Autodesk Inventor part; units mm, degrees
ref_plane "YZ Plane" through (0, 0, 0) normal (1, 0, 0) x (0, 1, 0)
ref_plane "XZ Plane" through (0, 0, 0) normal (0, 1, 0) x (-1, 0, 0)
ref_plane "XY Plane" through (0, 0, 0) normal (0, 0, 1) x (1, 0, 0)
sketch "Sketch1" plane through (0, 0, 0) normal (0, 0, 1) x (1, 0, 0)
  arc A0 (21.0123, -15.4044) -> (-20.0568, -16.8099) centre (-0.0744, 0.0265) ccw
  arc A1 (-1.3604, -38.9999) -> (3.8767, -38.8206) centre (1.1877, -36.8529) ccw
  line L0 (-1.3604, -38.9999) -> (-20.0568, -16.8099)
  line L1 (3.8767, -38.8206) -> (21.0123, -15.4044)
  point P0 (0, 0)
ref_plane "Work Plane1" through (21.0123, -15.4044, 0) normal (0.5906, 0.807, 0) x (-0.807, 0.5906, 0)
sketch "Sketch2" plane through (21.0123, -15.4044, 0) normal (0.5906, 0.807, 0) x (-0.807, 0.5906, 0)
  line L0 (1.0661, 2.0494) -> (-0.4231, 2.0494)
  line L1 (-0.4231, 2.0494) -> (-0.4231, -2.0661)
  line L2 (-0.4231, -2.0661) -> (1.0661, -2.0661)
  line L3 (1.0661, -2.0661) -> (1.0661, 2.0494)
  point P0 (26.054, 0)
sweep "Sweep1" add profiles "Sketch2" path "Sketch1"
properties part number "belt"
Work out the finished part from the listing and answer in its coordinate system (mm). A direction names the side the tool comes from. Round coordinates to 2 decimals unless told otherwise and drop trailing zeros. Write each loop counter-clockwise with the first axis right and the second up, starting at its lowest first coordinate (ties: lowest second). Pieces come first, ordered by that corner, then holes.
1) A cutting plane is placed at A-A on z = 0.35. Determine the outline of the cut face in (x, y).
2) Consider probe 1 along Y at (x, z) = (-6, -0.25); probe 2 along X at (y, z) = (-27, 1.2); probe 3 along Y at (x, z) = (7.5, 0.4). Determine where each line is inside the solid, lowest interval first.
3) Determine the mould class of faces 1 (the face through (-9.762, -27.373, -0.037)), 2 (the face through (20, -16, 2.049)), 3 (the face through (-1.813, 26.522, -0.037)) for opening direction X: pulls with the +X half, pulls with the -X half, needs draft (parallel to the pull), parting line crosses it, or undercut.
4) Flat-ended cylindrical pins translate along their axes: P1, Ø10, axis at x = 15.5, y = 10.5, coming from the +Z side; P2, Ø1, axis at y = 16.5, z = -1, coming from the -X side. Find the tip coordinate at first contact, or state that the pin passes through.
5) Which of the six approach directions +Z, -Z, +X, -X, +Y, -Y give full straight-line access (tool end or side, diameter ignored) to faces 4 (the face through (1.24, -39.12, 0.02)), 5 (the face through (-10.901, -28.333, 0.02))?
6) A cutting plane is placed at B-B on x = -5.5. Determine the outline of the cut face in (y, z).
7) A cutting plane is placed at C-C on y = 16. Determine the outline of the cut face in (x, z).
Entries:
1. outline: (-20.38, -17.08) - (-1.68, -39.27) arc R3.76 ccw to (4.22, -39.07) - (21.35, -15.65) arc R26.55 ccw (long way) to start; hole (-19.24, -16.12) - (-0.55, -38.31) arc R2.27 ccw to (3.02, -38.19) - (20.15, -14.77) arc R25.06 ccw (long way) to start
2. probe 1: y = -34.15 to -31.84, 24.38 to 25.91
2. probe 2: x = -12.02 to -10.08, 11.21 to 13.05
2. probe 3: y = -34.59 to -32.06, 23.92 to 25.48
3. face 1: undercut
3. face 2: needs draft
3. face 3: parting line crosses it
4. P1: passes through
4. P2: stops at x = -21.29
5. face 4: +Z, -Z
5. face 5: +Z, -Z, -X, -Y
6. outline: (-34.74, -2.07) - (-32.43, -2.07) - (-32.43, 2.05) - (-34.74, 2.05) - close; (24.5, -2.07) - (26.02, -2.07) - (26.02, 2.05) - (24.5, 2.05) - close
7. outline: (-21.29, -2.07) - (-19.39, -2.07) - (-19.39, 2.05) - (-21.29, 2.05) - close; (19.24, -2.07) - (21.14, -2.07) - (21.14, 2.05) - (19.24, 2.05) - close
